from build123d import *

# Parameters (mm, degrees)
PAD046_DEPTH    = 55
POCKET064_DEPTH = 147.675197


with BuildPart() as part:
    # Sketch126 → Pad046 (new body)
    with BuildSketch(Plane.XZ.offset(-27.5)):
        with BuildLine():
            ThreePointArc((-5.864892, -58.75), (-1.6403, -56.01044), (0, -51.25))
            Line((0, -51.25), (-17, -51.25))
            Line((-17, -51.25), (-36.926579, -64))
            Line((-36.926579, -64), (-27, -64))
            Line((-27, -64), (-5.864892, -58.75))
        make_face()
    extrude(amount=PAD046_DEPTH)

    # Sketch127 (on Face3 of Pad046) → Pocket064 (cut, through all)
    with BuildSketch(Plane(origin=(0, 0, -51.25), x_dir=(0, -1, 0), z_dir=(0, 0, 1))):
        with BuildLine():
            Line((-27.5, -17), (-27.5, -43))
            Line((-27.5, -43), (0, -43))
            Line((0, -43), (0, -17))
            Line((0, -17), (-15.050161, -17))
            ThreePointArc((-15.050161, -17), (-14.226455, -19.908295), (-12, -21.952695))
            Line((-12, -21.952695), (-15.2, -32.476953))
            ThreePointArc((-27.5, -17), (-24.05052, -26.884661), (-15.2, -32.476953))
        make_face()
    pocket064 = extrude(amount=-POCKET064_DEPTH, mode=Mode.SUBTRACT)

    # Mirrored003: Pocket064 across Sketch127 V_Axis
    add(pocket064.mirror(Plane(origin=(0, 0, -51.25), x_dir=(0, 0, 1), z_dir=(0, -1, 0))), mode=Mode.SUBTRACT)


with BuildPart() as part_1:
    # Body017 placement: moved
    add(part.part.moved(Location((32, 0, 0))))


solid = part_1.part
The model under review builds one solid part; all positions refer to its coordinate system, in mm. A direction names the side the tool comes from. Round coordinates to 2 decimals unless told otherwise and drop trailing zeros. Loops run counter-clockwise (first coordinate to the right, second up) from the corner with the lowest first, then second, coordinate; pieces in that order, holes last. Notation, with made-up numbers: (88.5, 23) - (109.5, 23) arc R21 cw to (109.5, 39) - close; hole circle Ø5 at (30, -6). An arc over 180 degrees is marked (long way). Use CSV: the item, a comma, the result in double quotes.
(1) Clearance check with flat-ended pins moving along their axes: P1, Ø3, axis at x = 19, y = 1.5, coming from the -Z side (3 decimals); P2, Ø5, axis at x = 9, y = 20, coming from the +Z side. State where each tip first meets the part, or that it passes through.
Working result:
P1,"stops at z = -60.895"
P2,"stops at z = -53.49"
(2) Take a section at A-A, the plane y = 13. Give the boundary of the cut face in (x, z).
Working result:
outline,"(6.76, -63.56) - (10.69, -62.59) - (10.69, -54) - (6.76, -56.52) - close; (15, -61.52) - (26.14, -58.75) arc R7.73 ccw to (32, -51.25) - (15, -51.25) - close"
(3) Machinability: for faces 4 (the flat face through (17.768, 0.385, -60.828)), 5 (the cylindrical face through (12.13, -14.25, -58.2)), 6 (the flat face through (6.03, -13.22, -60.21)), which of the approach directions +Z, -Z, +X, -X, +Y, -Y give a long, thin tool a straight path to every point of the face, cutting with its end or side? Answer none if there is none.
Working result:
face 4,"-Z, +X, +Y, -Y"
face 5,"+Z, -Z"
face 6,"+Z, -Z, -X"
(4) Take a section at B-B, the plane x = 9. Give the boundary of the cut face in (y, z).
Working result:
outline,"(-26.32, -63.01) - (-12.32, -63.01) - (-12.32, -55.09) - (-26.32, -55.09) - close; (12.32, -63.01) - (26.32, -63.01) - (26.32, -55.09) - (12.32, -55.09) - close"
(5) The part is to be moulded in two halves that separate along X. For faces 1 (the cylindrical face through (12.13, 14.25, -58.2)), 2 (the flat face through (3, -18, -64)), 3 (the cylindrical face through (7.204, 25.456, -60.369)), say which applies: pulls with the +X half, pulls with the -X half, needs draft (parallel to the pull), parting line crosses it, or undercut.
Working result:
face 1,"undercut"
face 2,"needs draft"
face 3,"pulls with the -X half"
(6) Take a section at C-C, the plane z = -59.75. Give the boundary of the cut face in (x, y).
Working result:
outline,"(1.72, -20.33) arc R15.89 ccw to (15, -27.5) - (22.11, -27.5) - (22.11, 27.5) - (15, 27.5) arc R15.89 ccw to (1.72, 20.33) - (1.72, 14.53) - (10.05, 12) arc R5.55 cw to (15, 15.05) - (15, -15.05) arc R5.55 cw to (10.05, -12) - (1.72, -14.53) - close"
(7) Take a section at D-D, the plane y = -4.5. Give the boundary of the cut face in (x, z).
Working result:
outline,"(15, -61.52) - (26.14, -58.75) arc R7.73 ccw to (32, -51.25) - (15, -51.25) - close"
(8) For line 1 (Y direction, x = 2, z = -61); line 2 (Y direction, x = 9, z = -61.5); line 3 (Z direction, x = 8.5, y = -21), list the stretches that pass through material, from the lowest coordinate up.
Working result:
line 1,"y = -20.75 to -14.45, 14.45 to 20.75"
line 2,"y = -26.32 to -12.32, 12.32 to 26.32"
line 3,"z = -63.13 to -55.41"
